Can you work these out from the model? Positions are in its coordinate system, mm. Face numbers are marked on the shaded views. A direction names the side the tool comes from. Round coordinates to 2 decimals unless told otherwise and drop trailing zeros. Loops run counter-clockwise (first coordinate to the right, second up) from the corner with the lowest first, then second, coordinate; pieces in that order, holes last.
```python
from build123d import *

# Parameters (mm, degrees)
SKETCH1_W           = 72
SKETCH1_H           = 75
SKETCH1_R           = 1.35
BOSS_EXTRUDE1_DEPTH = 6.35
BOSS_EXTRUDE2_DEPTH = 10
SKETCH3_W           = 58.5
SKETCH3_H           = 40
BOSS_EXTRUDE3_DEPTH = 2
FILLET1_R           = 5
SKETCH4_W           = 20
SKETCH4_H           = 20
BOSS_EXTRUDE4_DEPTH = 8.5
SKETCH5_W           = 7.5
SKETCH5_H           = 18.25
CUT_EXTRUDE1_DEPTH  = 18.5
FILLET2_R           = 0.5
FILLET3_R           = 2
FILLET4_R           = 2
CUT_EXTRUDE2_REACH  = 59.617
SKETCH6_W           = 13.5
SKETCH6_H           = 14
FILLET5_R           = 7
CUT_EXTRUDE3_REACH  = 59.617
SKETCH7_R           = 4.5


with BuildPart() as part:
    # Sketch1 → Boss-Extrude1 (new body)
    with BuildSketch(Plane.XY):
        Rectangle(SKETCH1_W, SKETCH1_H)
        with Locations((-32.83, 32.83)):
            Circle(SKETCH1_R, mode=Mode.SUBTRACT)
        with Locations((-32.83, -32.83)):
            Circle(SKETCH1_R, mode=Mode.SUBTRACT)
        with Locations((32.83, 32.83)):
            Circle(SKETCH1_R, mode=Mode.SUBTRACT)
        with Locations((32.83, -32.83)):
            Circle(SKETCH1_R, mode=Mode.SUBTRACT)
    extrude(amount=BOSS_EXTRUDE1_DEPTH)

    # Sketch2 → Boss-Extrude2 (add)
    with BuildSketch(Plane.XY.offset(6.35)):
        Polygon((-26.92, 32.5), (-28.92, 32.5), (-28.92, -35), (29.58, -35), (29.58, 32.5), (27.58, 32.5), (27.58, -32.5), (-26.92, -32.5), align=None)
    extrude(amount=BOSS_EXTRUDE2_DEPTH)

    # Sketch3 → Boss-Extrude3 (add)
    with BuildSketch(Plane.XY.offset(16.35)):
        with Locations((0.33, -15)):
            Rectangle(SKETCH3_W, SKETCH3_H)
    extrude(amount=-BOSS_EXTRUDE3_DEPTH)

    # Fillet1
    fillet1_edges = [part.edges().sort_by_distance(p)[0] for p in [
        (-26.92, 5, 15.35),
        (27.58, 5, 15.35),
    ]]
    fillet(fillet1_edges, radius=FILLET1_R)

    # Sketch4 → Boss-Extrude4 (add)
    with BuildSketch(Plane.XY.offset(16.35)):
        with Locations((15, -20)):
            Rectangle(SKETCH4_W, SKETCH4_H)
    extrude(amount=BOSS_EXTRUDE4_DEPTH)

    # Sketch5 → Cut-Extrude1 (cut)
    with BuildSketch(Plane(origin=(25, 0, 0), x_dir=(0, 0, -1), z_dir=(1, 0, 0))):
        with Locations((-20.1, -19.975)):
            Rectangle(SKETCH5_W, SKETCH5_H)
    extrude(amount=-CUT_EXTRUDE1_DEPTH, mode=Mode.SUBTRACT)

    # Fillet2
    fillet2_edges = [part.edges().sort_by_distance(p)[0] for p in [
        (15.75, -29.1, 23.85),
        (15.75, -10.85, 23.85),
    ]]
    fillet(fillet2_edges, radius=FILLET2_R)

    # Fillet3
    fillet3_edges = [part.edges().sort_by_distance(p)[0] for p in [
        (-28.92, -35, 11.35),
        (29.58, -35, 11.35),
        (36, -37.5, 3.175),
        (-36, -37.5, 3.175),
        (-36, 37.5, 3.175),
        (36, 37.5, 3.175),
    ]]
    fillet(fillet3_edges, radius=FILLET3_R)

    # Fillet4
    fillet4_edges = [part.edges().sort_by_distance(p)[0] for p in [
        (5, -10, 20.6),
        (5, -30, 20.6),
        (5, -20, 24.85),
    ]]
    fillet(fillet4_edges, radius=FILLET4_R)

    # Sketch6 → Cut-Extrude2 (cut, up to next)
    with BuildSketch(Plane.XY.offset(24.85), mode=Mode.PRIVATE) as cut_extrude2_sk1:
        with Locations((18.25, -20)):
            Rectangle(SKETCH6_W, SKETCH6_H)
    cut_extrude2_tool1 = extrude(cut_extrude2_sk1.sketch, amount=-CUT_EXTRUDE2_REACH, mode=Mode.PRIVATE) & part.part
    add(cut_extrude2_tool1.solids().sort_by_distance((18.25, -20, 24.85))[0], mode=Mode.SUBTRACT)

    # Fillet5
    fillet5_edges = [part.edges().sort_by_distance(p)[0] for p in [
        (11.5, -27, 24.35),
        (11.5, -13, 24.35),
    ]]
    fillet(fillet5_edges, radius=FILLET5_R - 0.0001)  # a hair under: the kernel refuses the full size

    # Sketch7 → Cut-Extrude3 (cut, up to next)
    with BuildSketch(Plane(origin=(0, 0, 0), x_dir=(-1, 0, 0), z_dir=(0, 0, -1)), mode=Mode.PRIVATE) as cut_extrude3_sk1:
        with Locations((-18.5, 18)):
            Circle(SKETCH7_R)
    cut_extrude3_tool1 = extrude(cut_extrude3_sk1.sketch, amount=-CUT_EXTRUDE3_REACH, mode=Mode.PRIVATE) & part.part
    # Sketch7 → Cut-Extrude3 (cut, up to next)
    with BuildSketch(Plane(origin=(0, 0, 0), x_dir=(-1, 0, 0), z_dir=(0, 0, -1)), mode=Mode.PRIVATE) as cut_extrude3_sk2:
        with Locations((0, 18)):
            Circle(SKETCH7_R)
    cut_extrude3_tool2 = extrude(cut_extrude3_sk2.sketch, amount=-CUT_EXTRUDE3_REACH, mode=Mode.PRIVATE) & part.part
    # Sketch7 → Cut-Extrude3 (cut, up to next)
    with BuildSketch(Plane(origin=(0, 0, 0), x_dir=(-1, 0, 0), z_dir=(0, 0, -1)), mode=Mode.PRIVATE) as cut_extrude3_sk3:
        with Locations((18.5, 18)):
            Circle(SKETCH7_R)
    cut_extrude3_tool3 = extrude(cut_extrude3_sk3.sketch, amount=-CUT_EXTRUDE3_REACH, mode=Mode.PRIVATE) & part.part
    # Sketch7 → Cut-Extrude3 (cut, up to next)
    with BuildSketch(Plane(origin=(0, 0, 0), x_dir=(-1, 0, 0), z_dir=(0, 0, -1)), mode=Mode.PRIVATE) as cut_extrude3_sk4:
        with Locations((-18.5, 0)):
            Circle(SKETCH7_R)
    cut_extrude3_tool4 = extrude(cut_extrude3_sk4.sketch, amount=-CUT_EXTRUDE3_REACH, mode=Mode.PRIVATE) & part.part
    # Sketch7 → Cut-Extrude3 (cut, up to next)
    with BuildSketch(Plane(origin=(0, 0, 0), x_dir=(-1, 0, 0), z_dir=(0, 0, -1)), mode=Mode.PRIVATE) as cut_extrude3_sk5:
        Circle(SKETCH7_R)
    cut_extrude3_tool5 = extrude(cut_extrude3_sk5.sketch, amount=-CUT_EXTRUDE3_REACH, mode=Mode.PRIVATE) & part.part
    # Sketch7 → Cut-Extrude3 (cut, up to next)
    with BuildSketch(Plane(origin=(0, 0, 0), x_dir=(-1, 0, 0), z_dir=(0, 0, -1)), mode=Mode.PRIVATE) as cut_extrude3_sk6:
        with Locations((18.5, 0)):
            Circle(SKETCH7_R)
    cut_extrude3_tool6 = extrude(cut_extrude3_sk6.sketch, amount=-CUT_EXTRUDE3_REACH, mode=Mode.PRIVATE) & part.part
    # Sketch7 → Cut-Extrude3 (cut, up to next)
    with BuildSketch(Plane(origin=(0, 0, 0), x_dir=(-1, 0, 0), z_dir=(0, 0, -1)), mode=Mode.PRIVATE) as cut_extrude3_sk7:
        with Locations((0, -18)):
            Circle(SKETCH7_R)
    cut_extrude3_tool7 = extrude(cut_extrude3_sk7.sketch, amount=-CUT_EXTRUDE3_REACH, mode=Mode.PRIVATE) & part.part
    # Sketch7 → Cut-Extrude3 (cut, up to next)
    with BuildSketch(Plane(origin=(0, 0, 0), x_dir=(-1, 0, 0), z_dir=(0, 0, -1)), mode=Mode.PRIVATE) as cut_extrude3_sk8:
        with Locations((18.5, -18)):
            Circle(SKETCH7_R)
    cut_extrude3_tool8 = extrude(cut_extrude3_sk8.sketch, amount=-CUT_EXTRUDE3_REACH, mode=Mode.PRIVATE) & part.part
    # Sketch7 → Cut-Extrude3 (cut, up to next)
    with BuildSketch(Plane(origin=(0, 0, 0), x_dir=(-1, 0, 0), z_dir=(0, 0, -1)), mode=Mode.PRIVATE) as cut_extrude3_sk9:
        with Locations((-18.5, -18)):
            Circle(SKETCH7_R)
    cut_extrude3_tool9 = extrude(cut_extrude3_sk9.sketch, amount=-CUT_EXTRUDE3_REACH, mode=Mode.PRIVATE) & part.part
    add(cut_extrude3_tool1.solids().sort_by_distance((18.5, 18, 0))[0], mode=Mode.SUBTRACT)
    add(cut_extrude3_tool2.solids().sort_by_distance((0, 18, 0))[0], mode=Mode.SUBTRACT)
    add(cut_extrude3_tool3.solids().sort_by_distance((-18.5, 18, 0))[0], mode=Mode.SUBTRACT)
    add(cut_extrude3_tool4.solids().sort_by_distance((18.5, 0, 0))[0], mode=Mode.SUBTRACT)
    add(cut_extrude3_tool5.solids().sort_by_distance((0, 0, 0))[0], mode=Mode.SUBTRACT)
    add(cut_extrude3_tool6.solids().sort_by_distance((-18.5, 0, 0))[0], mode=Mode.SUBTRACT)
    add(cut_extrude3_tool7.solids().sort_by_distance((0, -18, 0))[0], mode=Mode.SUBTRACT)
    add(cut_extrude3_tool8.solids().sort_by_distance((-18.5, -18, 0))[0], mode=Mode.SUBTRACT)
    add(cut_extrude3_tool9.solids().sort_by_distance((18.5, -18, 0))[0], mode=Mode.SUBTRACT)


solid = part.part
```
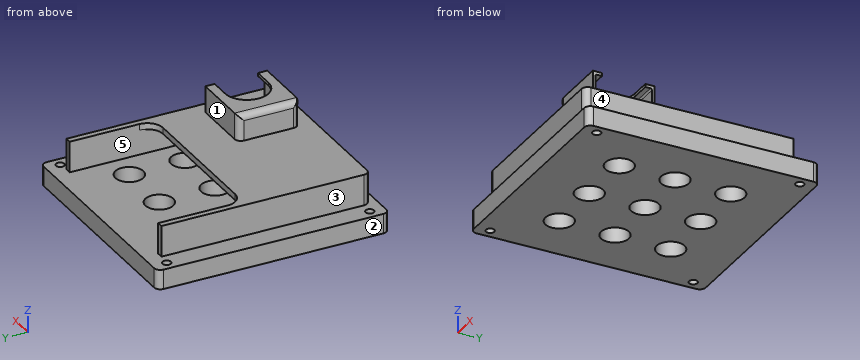
(1) Suppose I cut it at C-C (z = 5.25). Give the number of separate pieces and of enclosed holes in the cut face, then the cut area to 3 significant figures.
(2) Suppose I cut it at B-B (x = -32.83). Write out the boundary of the cut face in (y, z).
(3) For pin 1 (7.5 mm diameter, centred on x = 17, z = 21, fed in from -Y); pin 2 (8 mm diameter, centred on x = -18.5, y = 4, fed in from +Z); pin 3 (3 mm diameter, centred on y = -17.5, z = 20.5, fed in from -X), each with a flat end and sliding along its axis, tell me the tip position at first contact or that it passes through.
(4) Suppose I cut it at D-D (y = 25). Write out the boundary of the cut face in (x, z), then the cut area to 3 significant figures.
(5) If I drill on line 1 (Z direction, x = 11.5, y = -16.5); line 2 (Y direction, x = 18.5, z = 5); line 3 (Y direction, x = 32.83, z = 4.5), over which ranges is the centre line in solid material (lowest first)?
(6) We'd pull the mould along Y, two halves only. Please class the marked faces 1 and 2: released by +Y, released by -Y, zero draft, split by the parting line, or undercut.
(7) Suppose I cut it at A-A (y = 0). Write out the boundary of the cut face in (x, z).
(8) Which directions (+Z, -Z, +X, -X, +Y, -Y) give clear straight access to the entire face, cutting with the end or side of a thin tool? Please do the marked faces 3, 4 and 5.
Check result:
1. separate pieces: 1
1. enclosed holes: 13
1. area: 4,800 mm2
2. outline: (-37.5, 0) - (-34.18, 0) - (-34.18, 6.35) - (-37.5, 6.35) - close; (-31.48, 0) - (31.48, 0) - (31.48, 6.35) - (-31.48, 6.35) - close; (34.18, 0) - (37.5, 0) - (37.5, 6.35) - (34.18, 6.35) - close
3. pin 1: stops at y = -30
3. pin 2: stops at z = 16.35
3. pin 3: stops at x = 5
4. outline: (-36, 0) - (36, 0) - (36, 6.35) - (29.58, 6.35) - (29.58, 16.35) - (27.58, 16.35) - (27.58, 6.35) - (-26.92, 6.35) - (-26.92, 16.35) - (-28.92, 16.35) - (-28.92, 6.35) - (-36, 6.35) - close
4. area: 497 mm2
5. line 1: z = 0 to 6.35, 14.35 to 16.35, 23.85 to 24.85
5. line 2: y = -37.5 to -22.5, -13.5 to -4.5, 4.5 to 13.5, 22.5 to 37.5
5. line 3: y = -37.5 to -34.18, -31.48 to 31.48, 34.18 to 37.5
6. face 1: released by +Y
6. face 2: zero draft
7. outline: (-36, 0) - (-23, 0) - (-23, 6.35) - (-26.92, 6.35) - (-26.92, 14.35) - (27.58, 14.35) - (27.58, 6.35) - (23, 6.35) - (23, 0) - (36, 0) - (36, 6.35) - (29.58, 6.35) - (29.58, 16.35) - (-28.92, 16.35) - (-28.92, 6.35) - (-36, 6.35) - close; (-14, 0) - (-4.5, 0) - (-4.5, 6.35) - (-14, 6.35) - close; (4.5, 0) - (14, 0) - (14, 6.35) - (4.5, 6.35) - close
8. face 3: +Z, -X, +Y, -Y
8. face 4: +Z, +X, +Y, -Y
8. face 5: +Y
